Work out the finished part from the listing and answer in its coordinate system (mm). A direction names the side the tool comes from. Round coordinates to 2 decimals unless told otherwise and drop trailing zeros. Write each loop counter-clockwise with the first axis right and the second up, starting at its lowest first coordinate (ties: lowest second). Pieces come first, ordered by that corner, then holes.
1. Find section B-B (y = 6.25). Write down the section's boundary in (x, z), and give its area (3 significant figures).
2. A tool of negligible diameter and unlimited length cuts with its end or side. For faces 1 (the face through (0, 0, 800)), 2 (the face through (0, -2.5, -19)), 3 (the face through (0, 2.5, -19)), from which of +Z, -Z, +X, -X, +Y, -Y can it reach the whole face along a straight path? Write none if from no direction.
3. Flat-ended cylindrical pins translate along their axes: pin 1 Ø2.5 at (x, y) = (-9, 5) entering from -Z; pin 2 Ø8 at (x, y) = (0, 4.5) entering from -Z; pin 3 Ø3 at (y, z) = (-2, 62) entering from -X; pin 4 Ø1 at (x, z) = (12, 507.5) entering from -Y. Find the tip coordinate at first contact, or state that the pin passes through.
4. Straight lines are drawn through the part: probe 1 along Z at (x, y) = (15, 5.75); probe 2 along Y at (x, z) = (-11.5, 176); probe 3 along Z at (x, y) = (-18, 1.5). For each, find the intervals that lie inside material, in ascending order.
```python
from build123d import *

# Parameters (mm, degrees)
F0_W     = 40
F0_H     = 20
F1_DEPTH = 800
F2_R     = 9.99999
F4_DEPTH = 2.5


# Not quite as in the source:
# - a fillet or chamfer is up to 0.001 mm smaller than in the source, because OpenCascade refuses the exact size


with BuildPart() as f1:
    # F0 (on Top) → F1 (new body)
    with BuildSketch(Plane.XY):
        Rectangle(F0_W, F0_H)
    extrude(amount=F1_DEPTH)

    # F2 (radius 10 in the source; OpenCascade refuses exactly that, so slightly less here)
    f2_edges = [f1.edges().sort_by_distance(p)[0] for p in [
        (20, -10, 400),
        (20, 10, 400),
        (-20, -10, 400),
        (-20, 10, 400),
    ]]
    fillet(f2_edges, radius=F2_R)

    # F3 (on Front) → F4 (join, symmetric)
    with BuildSketch(Plane.XZ):
        Polygon((19.9430335092, 0), (-20.0569664908, 0), (0, -50), align=None)
    extrude(amount=F4_DEPTH, both=True)


solid = f1.part
```
Worked answers:
1. outline: (-17.81, 0) - (17.81, 0) - (17.81, 800) - (-17.81, 800) - close
1. area: 28,500 mm2
2. face 1: +Z, +X, -X, +Y, -Y
2. face 2: -Z, +X, -X, -Y
2. face 3: -Z, +X, -X, +Y
3. pin 1: stops at z = 0
3. pin 2: stops at z = -50
3. pin 3: stops at x = -19.99
3. pin 4: stops at y = -9.89
4. probe 1: z = 0 to 800
4. probe 2: y = -9.89 to 9.89
4. probe 3: z = -5.13 to 800
